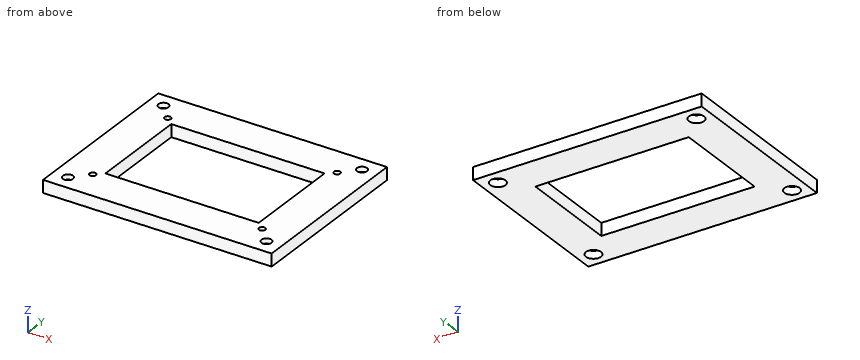
Autodesk Inventor part; units mm, degrees
ref_plane "YZ Plane" through (0, 0, 0) normal (1, 0, 0) x (0, 1, 0)
ref_plane "XZ Plane" through (0, 0, 0) normal (0, 1, 0) x (-1, 0, 0)
ref_plane "XY Plane" through (0, 0, 0) normal (0, 0, 1) x (1, 0, 0)
sketch "Sketch1" plane through (0, 0, 0) normal (0, 0, 1) x (1, 0, 0)
  line L0 (-30.5, -20) -> (30.5, -20)
  line L1 (30.5, -20) -> (30.5, 20)
  line L2 (30.5, 20) -> (-30.5, 20)
  line L3 (-30.5, 20) -> (-30.5, -20)
  line L4 (-30.5, -20) -> (30.5, 20) construction
  line L5 (30.5, -20) -> (-30.5, 20) construction
  line L6 (-45.5, -35) -> (45.5, -35)
  line L7 (45.5, -35) -> (45.5, 35)
  line L8 (45.5, 35) -> (-45.5, 35)
  line L9 (-45.5, 35) -> (-45.5, -35)
  line L10 (-45.5, -35) -> (45.5, 35) construction
  line L11 (45.5, -35) -> (-45.5, 35) construction
  point P0 (0, 0)
  dimension "d0" = 61
  dimension "d1" = 40
  dimension "d2" = 15
  dimension "d3" = 15
extrude "Rim" add sketch "Sketch1" along normal blind 5
sketch "Sketch2" plane through (0, 0, 5) normal (0, 0, 1) x (1, 0, 0)
  line L0 (-33.7, -22.765) -> (33.7, -22.765) construction
  line L1 (33.7, -22.765) -> (33.7, 22.765) construction
  line L2 (33.7, 22.765) -> (-33.7, 22.765) construction
  line L3 (-33.7, 22.765) -> (-33.7, -22.765) construction
  line L4 (-33.7, -22.765) -> (33.7, 22.765) construction
  line L5 (33.7, -22.765) -> (-33.7, 22.765) construction
  circle A0 centre (33.7, 22.765) radius 1.25
  line L6 (0, 22.765) -> (0, -22.765) construction
  line L7 (-30.5, -20) -> (-30.5, 20)
  line L8 (-30.5, 0) -> (33.7, 0) construction
  circle A1 centre (-33.7, 22.765) radius 1.25
  circle A2 centre (33.7, -22.765) radius 1.25
  circle A3 centre (-33.7, -22.765) radius 1.25
  point P0 (0, 0)
  dimension "d6" = 67.4
  dimension "d7" = 45.53
  dimension "d8" = 2.5
extrude "Pegs" cut sketch "Sketch2" against normal blind 3
sketch "Sketch4" plane through (0, 0, 0) normal (0, 0, -1) x (-1, 0, 0)
  circle A0 centre (-39.5, 29) radius 2
  circle A1 centre (39.5, 29) radius 2
  circle A2 centre (39.5, -29) radius 2
  circle A3 centre (-39.5, -29) radius 2
  point P0 (0, 0)
extrude "Bolt Holes" cut sketch "Sketch4" against normal up to next
sketch "For Construction" plane through (0, 0, 5) normal (0, 0, 1) x (1, 0, 0)
  circle A0 centre (33.7, -22.765) radius 1.25
  circle A1 centre (39.5, -29) radius 2
  point P0 (0, 0)
  point P1 (34.95, -22.765)
  point P2 (37.901, -27.7986)
  dimension "d19" = 5.2656
ref_plane "Work Plane2" through (-30.5, 0, 0) normal (0, 1, 0) x (1, 0, 0)
sketch "Sketch13" plane through (0, 0, 0) normal (0, 0, -1) x (-1, 0, 0)
  circle A0 centre (-39.5, -29) radius 3
  circle A1 centre (-39.5, -29) radius 2
  line L0 (45.5, -35) -> (-45.5, -35)
  line L1 (0, -35) -> (0, -20) construction
  line L2 (-30.5, -20) -> (30.5, -20)
  line L3 (-27.3467, 0) -> (-45.5, 0) construction
  line L4 (-45.5, -35) -> (-45.5, 35)
  line L5 (-45.5, -35) -> (-45.5, 35)
  circle A2 centre (-39.5, 29) radius 3
  circle A3 centre (39.5, -29) radius 3
  circle A4 centre (39.5, 29) radius 3
  point P0 (0, 0)
  dimension "d42" = 6
extrude "Bolt heads" cut sketch "Sketch13" against normal blind 3
properties part number "Joystickboard Holder"
Read the model definition and answer for the solid it produces. Units are mm, in the model's axes. Round coordinates to 2 decimals unless told otherwise and drop trailing zeros. Write each loop counter-clockwise with the first axis right and the second up, starting at its lowest first coordinate (ties: lowest second). Pieces come first, ordered by that corner, then holes.
1. The part is cut by section C-C, the plane z = 1.05. Determine the outline of the cut face in (x, y), then the cut area to 3 significant figures.
2. The part is cut by section B-B, the plane x = 39.5. Determine the outline of the cut face in (y, z).
3. Given pin 1 Ø1.5 at (x, y) = (33.7, -22.765) entering from +Z; pin 2 Ø4.5 at (x, y) = (39.5, 29) entering from -Z, each flat-ended and moving along its own axis, determine where each tip first touches the part or whether it passes through.
4. The part is cut by section A-A, the plane y = -29. Determine the outline of the cut face in (x, z), then the cut area to 3 significant figures.
5. Straight lines are drawn through the part: L1, parallel to Y at x = 33.7, z = 3.6 (3 decimals); L2, parallel to Y at x = 39.5, z = 3.4; L3, parallel to Y at x = -23, z = 2.2. For each, find the intervals that lie inside material, in ascending order.
6. The part is cut by section D-D, the plane x = -1.5. Determine the outline of the cut face in (y, z), then the cut area to 3 significant figures.
Values:
1. outline: (-45.5, -35) - (45.5, -35) - (45.5, 35) - (-45.5, 35) - close; hole circle Ø6 at (-39.5, -29); hole circle Ø6 at (-39.5, 29); hole (-30.5, -20) - (30.5, -20) - (30.5, 20) - (-30.5, 20) - close; hole circle Ø6 at (39.5, -29); hole circle Ø6 at (39.5, 29)
1. area: 3,820 mm2
2. outline: (-35, 0) - (-32, 0) - (-32, 3) - (-31, 3) - (-31, 5) - (-35, 5) - close; (-27, 3) - (-26, 3) - (-26, 0) - (26, 0) - (26, 3) - (27, 3) - (27, 5) - (-27, 5) - close; (31, 3) - (32, 3) - (32, 0) - (35, 0) - (35, 5) - (31, 5) - close
3. pin 1: stops at z = 2
3. pin 2: stops at z = 3
4. outline: (-45.5, 0) - (-42.5, 0) - (-42.5, 3) - (-41.5, 3) - (-41.5, 5) - (-45.5, 5) - close; (-37.5, 3) - (-36.5, 3) - (-36.5, 0) - (36.5, 0) - (36.5, 3) - (37.5, 3) - (37.5, 5) - (-37.5, 5) - close; (41.5, 3) - (42.5, 3) - (42.5, 0) - (45.5, 0) - (45.5, 5) - (41.5, 5) - close
4. area: 403 mm2
5. L1: y = -35 to -24.015, -21.515 to 21.515, 24.015 to 35
5. L2: y = -35 to -31, -27 to 27, 31 to 35
5. L3: y = -35 to -20, 20 to 35
6. outline: (-35, 0) - (-20, 0) - (-20, 5) - (-35, 5) - close; (20, 0) - (35, 0) - (35, 5) - (20, 5) - close
6. area: 150 mm2
